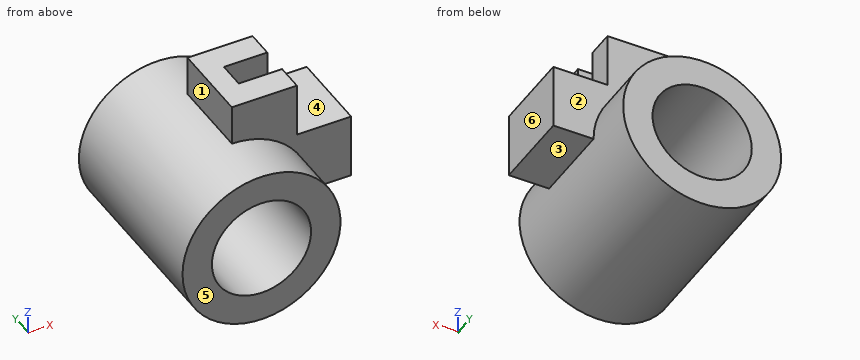
Autodesk Inventor part; units mm, degrees
ref_plane "YZ Plane" through (0, 0, 0) normal (1, 0, 0) x (0, 1, 0)
ref_plane "XZ Plane" through (0, 0, 0) normal (0, 1, 0) x (-1, 0, 0)
ref_plane "XY Plane" through (0, 0, 0) normal (0, 0, 1) x (1, 0, 0)
sketch "Boceto1" plane through (0, 0, 0) normal (0, 1, 0) x (-1, 0, 0)
  circle A0 centre (0, 0) radius 9.154
  circle A1 centre (0, 0) radius 14.5725
extrude "Extrusión1" add sketch "Boceto1" along normal mid plane 35
sketch "Boceto2" plane through (0, 0, 0) normal (0, 1, 0) x (-1, 0, 0)
  line L0 (-12, 0) -> (-22, 0)
  line L1 (-22, 0) -> (-22, 12)
  line L2 (-22, 12) -> (-12, 12)
  line L3 (-12, 12) -> (-12, 22)
  line L4 (-12, 22) -> (0, 22)
  line L5 (0, 22) -> (0, 12)
  arc A0 (0, 12) -> (-12, 0) centre (0, 0) ccw
  line L6 (0, 0) -> (0, 23.3606) construction
  line L7 (0, 0) -> (-38.6088, 0) construction
  point P0 (0, 17)
  dimension "d4" = 10
  dimension "d5" = 12
  dimension "d6" = 10
  dimension "d7" = 12
  dimension "d10" = 10
  dimension "d11" = 10
extrude "Extrusión2" add sketch "Boceto2" along normal mid plane 15
sketch "Boceto3" plane through (0, 7.5, 22) normal (0, 0, 1) x (1, 0, 0)
  line L0 (4, -5) -> (12, -5)
  line L1 (12, -5) -> (12, -10)
  line L2 (12, -10) -> (4, -10)
  line L3 (4, -10) -> (4, -5)
  line L4 (12, -15) -> (12, 0)
  line L5 (12, -15) -> (0, -15)
  point P0 (0, -7.5)
  dimension "d8" = 5
  dimension "d9" = 5
  dimension "d14" = 8
extrude "Extrusión3" cut sketch "Boceto3" against normal blind 10
sketch "Boceto5" plane through (12, 7.5, 12) normal (0, 0, 1) x (1, 0, 0)
  point P0 (-12, -7.5)
properties part number "Sujetador"
Geometry: final body of the model. Coordinates: model frame, mm. Face numbers are marked on the shaded views. A direction names the side the tool comes from. Round coordinates to 2 decimals unless told otherwise and drop trailing zeros. Order: outer loops, then holes, each group sorted by start corner. A loop starts at its lowest first (then second) coordinate and runs counter-clockwise, first axis right, second up. Notation, with made-up numbers: (73.25, 60.5) -> (84.25, 60.5) arc R32 cw to (84.25, 94.5) -> close; hole circle Ø10 at (41.25, 34). An arc over 180 degrees is marked (long way). Use one line per item in the form item = value.
(1) Ray query, probe 1 along Z at (x, y) = (12.5, -6.5); probe 2 along X at (y, z) = (2.5, -7); probe 3 along Z at (x, y) = (-0.5, -12.5). Return the intervals inside material, ascending. Write a range as [from, to].
Results list:
probe_1 = [-7.49, 12]
probe_2 = [-12.78, -5.9], [5.9, 12.78]
probe_3 = [-14.56, -9.14], [9.14, 14.56]
(2) Section B-B on x = 7.5. Return loops of the section in (y, z).
Results list:
outline = (-17.5, -12.49) -> (17.5, -12.49) -> (17.5, -5.25) -> (-17.5, -5.25) -> close; (-17.5, 5.25) -> (17.5, 5.25) -> (17.5, 12.49) -> (7.5, 12.49) -> (7.5, 22) -> (2.5, 22) -> (2.5, 12) -> (-2.5, 12) -> (-2.5, 22) -> (-7.5, 22) -> (-7.5, 12.49) -> (-17.5, 12.49) -> close
(3) Access query for the marked faces 1, 2 and 3. Directions: +Z, -Z, +X, -X, +Y, -Y. A direction counts if a zero-diameter tool reaches every point of the face in a straight line with its end or side. Return the directions, or none.
Results list:
face_1 = +Z, -X, +Y, -Y
face_2 = +Z, +X, +Y
face_3 = -Z, +X, +Y, -Y
(4) Section A-A on y = 1.5. Return loops of the section in (x, z) (1 decimal), and give its area (3 significant figures).
Results list:
outline = (0, 14.6) arc R14.6 ccw (long way) to (14.6, 0) -> (22, 0) -> (22, 12) -> (4, 12) -> (4, 22) -> (0, 22) -> close; hole circle Ø18.3 at (0, 0)
area = 541 mm^2
(5) Draft query along Y for the marked faces 4, 5 and 6. Return one class per face: pulls with the +Y half, pulls with the -Y half, needs draft (parallel to the pull), parting line crosses it, or undercut.
Results list:
face_4 = undercut
face_5 = pulls with the -Y half
face_6 = needs draft
(6) Section D-D on y = -4. Return loops of the section in (x, z) (1 decimal), and give its area (3 significant figures).
Results list:
outline = (0, 14.6) arc R14.6 ccw (long way) to (14.6, 0) -> (22, 0) -> (22, 12) -> (12, 12) -> (12, 22) -> (0, 22) -> close; hole circle Ø18.3 at (0, 0)
area = 621 mm^2
(7) First-contact query: pin 1 Ø2.5 at (y, z) = (-4, 19) entering from +X; pin 2 Ø16.5 at (x, y) = (14.5, 0.5) entering from +Z; pin 3 Ø6 at (x, y) = (19, 2) entering from -Z; pin 4 Ø12 at (x, y) = (11, -13) entering from -Z. Flat tips, straight axial feed; report the tip coordinate or a pass-through.
Results list:
pin_1 = 12
pin_2 = 22
pin_3 = 0
pin_4 = -13.69
(8) Section C-C on z = -4. Return loops of the section in (x, y).
Results list:
outline = (-14.01, -17.5) -> (-8.23, -17.5) -> (-8.23, 17.5) -> (-14.01, 17.5) -> close; (8.23, -17.5) -> (14.01, -17.5) -> (14.01, 17.5) -> (8.23, 17.5) -> close
